For this review, take the finished solid that the model builds, in its own axes (mm). Round coordinates to 2 decimals unless told otherwise and drop trailing zeros. Loops run counter-clockwise (first coordinate to the right, second up) from the corner with the lowest first, then second, coordinate; pieces in that order, holes last. Notation, with made-up numbers: M 20.25,15.5 L 28.25,15.5 A24 ccw 28.25,44.5 Z; hole C -23.75,-36 d7. An arc over 180 degrees is marked long. Write item = value, one per line. Start each with the question number.
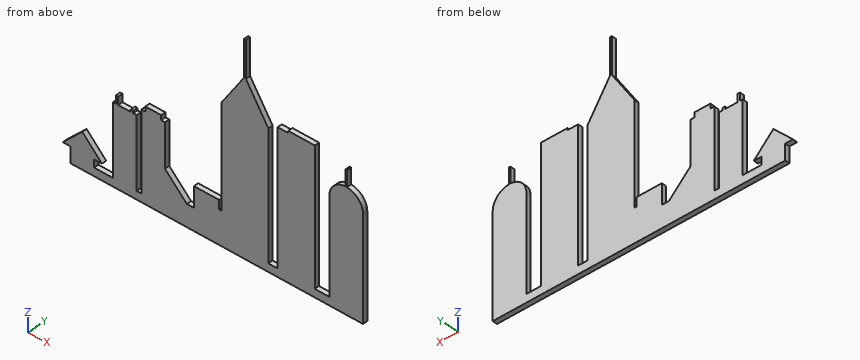
```python
from build123d import *

# Parameters (mm, degrees)
F0_W     = 12.0587127507
F0_H     = 5.1275454462
F0_W_2   = 3.073014915
F0_W_3   = 1.5
F0_H_2   = 5
F0_W_4   = 5.8694817126
F0_H_3   = 1.5
F0_W_5   = 10
F0_H_4   = 3
F0_W_6   = 9.2557147145
F1_DEPTH = 3


with BuildPart() as f1:
    # F0 (on Front) → F1 (new body)
    with BuildSketch(Plane.XZ):
        Polygon((-85.9764102697, -32.9992154241), (-85.9764102697, -42.9992154241), (-70.9764102697, -42.9992154241), (-70.9764102697, -37.8716699779), (-70.9764102697, -32.9992154241), (-65.9764102697, -32.9992154241), (-78.4764102697, -20.4992154241), (-90.9764102697, -32.9992154241), align=None)
        with Locations((-64.9470538944, -40.435442701)):
            Rectangle(F0_W, F0_H)
        Polygon((-58.9176975191, -37.8716699779), (-58.9176975191, -42.9992154241), (-43.9176975191, -42.9992154241), (-43.9176975191, -37.8716699779), (-43.9176975191, 7.0007845759), (-46.1646348834, 7.0007845759), (-47.6646348834, 7.0007845759), (-55.679722935, 7.0007845759), (-57.179722935, 7.0007845759), (-58.9176975191, 7.0007845759), align=None)
        with Locations((-42.3811900616, -40.435442701)):
            Rectangle(F0_W_2, F0_H)
        Polygon((-40.8446826041, -37.8716699779), (-40.8446826041, -42.9992154241), (-25.8446826041, -42.9992154241), (-25.8446826041, -15.4992154241), (-25.8446826041, 12.0007845759), (-28.3446826041, 12.0007845759), (-38.3446826041, 12.0007845759), (-40.8446826041, 12.0007845759), align=None)
        Polygon((-25.8446826041, -15.4992154241), (-25.8446826041, -42.9992154241), (39.9925373495, -42.9992154241), (39.9925373495, -37.8716699779), (39.9925373495, 42.0007845759), (25.0529701523, 42.0007845759), (10.1134029552, 42.0007845759), (10.1134029552, -21.9735670835), (8.6134029552, -21.9735670835), (8.6134029552, -16.3298398256), (-7.4147884734, -16.3298398256), (-7.4147884734, -29.1975438595), (-11.9297718629, -29.1975438595), align=None)
        with Locations((-56.429722935, 9.5007845759)):
            Rectangle(F0_W_3, F0_H_2)
        with Locations((42.9272782058, -40.435442701)):
            Rectangle(F0_W_4, F0_H)
        with Locations((-46.9146348834, 7.7507845759)):
            Rectangle(F0_W_3, F0_H_3)
        Polygon((45.862019062, -37.8716699779), (45.862019062, -42.9992154241), (69.5656836033, -42.9992154241), (69.5656836033, -37.8716699779), (69.5656836033, 47.0007845759), (52.6344925165, 47.0007845759), (52.6344925165, 45.7507845759), (45.862019062, 45.7507845759), align=None)
        with Locations((-33.3446826041, 13.5007845759)):
            Rectangle(F0_W_5, F0_H_4)
        with Locations((74.1935409606, -40.435442701)):
            Rectangle(F0_W_6, F0_H)
        Polygon((25.0529701523, 42.0007845759), (39.9925373495, 42.0007845759), (25.6491004298, 64.0628009761), (25.0529701523, 64.979724586), align=None)
        with BuildLine():
            Line((78.8213983178, -37.8716699779), (78.8213983178, -42.9992154241))
            Line((78.8213983178, -42.9992154241), (100.2675741911, -42.9992154241))
            Line((100.2675741911, -42.9992154241), (100.2675741911, 21.5343244148))
            Line((100.2675741911, 21.5343244148), (100.2675741911, 22.4990192801))
            ThreePointArc((100.2675741911, 22.4990192801), (97.140766726, 29.6004569802), (90.0444862545, 32.7389511733))
            ThreePointArc((90.0444862545, 32.7389511733), (89.5444862545, 32.7506028116), (89.0444862545, 32.7389511733))
            ThreePointArc((89.0444862545, 32.7389511733), (81.9482057829, 29.6004569802), (78.8213983178, 22.4990192801))
            Line((78.8213983178, 22.4990192801), (78.8213983178, 21.5343244148))
            Line((78.8213983178, 21.5343244148), (78.8213983178, -37.8716699779))
        make_face()
        Polygon((10.1134029552, 42.0007845759), (25.0529701523, 42.0007845759), (25.0529701523, 64.979724586), (24.3911507636, 63.9617628318), align=None)
        Polygon((25.0529701523, 64.979724586), (25.6491004298, 64.0628009761), (25.6491004298, 87.0592445135), (25.0529701523, 87.0592445135), align=None)
        Polygon((24.3911507636, 63.9617628318), (25.0529701523, 64.979724586), (25.0529701523, 87.0592445135), (24.3911507636, 87.0592445135), align=None)
        with BuildLine():
            Line((100.2675741911, 22.4990192801), (100.2675741911, 21.5343244148))
            ThreePointArc((100.2675741911, 21.5343244148), (100.2784172186, 22.0166718474), (100.2675741911, 22.4990192801))
        make_face()
        with BuildLine():
            ThreePointArc((78.8213983178, 22.4990192801), (78.8105552903, 22.0166718474), (78.8213983178, 21.5343244148))
            Line((78.8213983178, 21.5343244148), (78.8213983178, 22.4990192801))
        make_face()
        with BuildLine():
            ThreePointArc((89.0444862545, 32.7389511733), (89.5444862545, 32.7506028116), (90.0444862545, 32.7389511733))
            Line((90.0444862545, 32.7389511733), (90.0444862545, 42.7506028116))
            Line((90.0444862545, 42.7506028116), (89.0444862545, 42.7506028116))
            Line((89.0444862545, 42.7506028116), (89.0444862545, 32.7389511733))
        make_face()
    extrude(amount=F1_DEPTH)


solid = f1.part
```
(1) Add section B-B on z = 36. Write out the cut boundary in (x, y), and give its area (3 significant figures).
(2) Add section A-A on z = 18.5. Write out the cut boundary in (x, y).
(3) For pin 1 Ø1.1 at (x, y) = (89.5, -2) entering from +Z; pin 2 Ø0.9 at (y, z) = (-1.5, -34.5) entering from +X; pin 3 Ø1.5 at (y, z) = (-2, 74.5) entering from -X, all flat-tipped, find the tip position at first contact; note any pin that passes through.
(4) Wall thickness on L1, parallel to X at y = -1, z = -2; L2, parallel to X at y = -0.7, z = 21.5; L3, parallel to X at y = -2.1, z = 37: over which ranges is each line inside the solid? List them lowest first.
(5) Add section D-D on z = -24. Write out the cut boundary in (x, y), and give its area (3 significant figures).
(6) Add section C-C on x = -2. Write out the cut boundary in (y, z).
Answer sheet:
q1.outline = M 10.11,-3 L 39.99,-3 L 39.99,0 L 10.11,0 Z; M 45.86,-3 L 69.57,-3 L 69.57,0 L 45.86,0 Z; M 89.04,-3 L 90.04,-3 L 90.04,0 L 89.04,0 Z
q1.area = 164 mm²
q2.outline = M 10.11,-3 L 39.99,-3 L 39.99,0 L 10.11,0 Z; M 45.86,-3 L 69.57,-3 L 69.57,0 L 45.86,0 Z; M 78.82,-3 L 100.27,-3 L 100.27,0 L 78.82,0 Z
q3.pin_1 = 42.75
q3.pin_2 = 100.27
q3.pin_3 = 24.39
q4.L1 = -58.92 to -43.92, -40.84 to -25.84, 10.11 to 39.99, 45.86 to 69.57, 78.82 to 100.27
q4.L2 = 10.11 to 39.99, 45.86 to 69.57, 78.82 to 100.27
q4.L3 = 10.11 to 39.99, 45.86 to 69.57, 89.04 to 90.04
q5.outline = M -81.98,-3 L -74.98,-3 L -74.98,0 L -81.98,0 Z; M -58.92,-3 L -43.92,-3 L -43.92,0 L -58.92,0 Z; M -40.84,-3 L -17.21,-3 L -17.21,0 L -40.84,0 Z; M -7.41,-3 L 39.99,-3 L 39.99,0 L -7.41,0 Z; M 45.86,-3 L 69.57,-3 L 69.57,0 L 45.86,0 Z; M 78.82,-3 L 100.27,-3 L 100.27,0 L 78.82,0 Z
q5.area = 415 mm²
q6.outline = M -3,-43 L 0,-43 L 0,-16.33 L -3,-16.33 Z
